CAD build for the part. Positions are in the model's coordinates, mm. A direction names the side the tool comes from. Coordinates: 2 decimals unless noted, no trailing zeros. Order: outer loops, then holes, each group sorted by start corner. A loop starts at its lowest first (then second) coordinate and runs counter-clockwise, first axis right, second up. Notation, with made-up numbers: (23, -35.5) - (58, -35.5) arc R19 cw to (58, -23.5) - close; hole circle Ø8 at (68, -12). An arc over 180 degrees is marked (long way). Write each question's results on one line, items separated by ' | '. Start each with the question number.
Q1. Wall check: probe 1 along X at (y, z) = (-33.5, 0.25); probe 2 along Y at (x, z) = (32, -1); probe 3 along X at (y, z) = (-19.5, -2.5). Give the ranges that are in metal, low to high.
Q2. Which spindle directions (+Z, -Z, +X, -X, +Y, -Y) get a long thin tool onto all of the face, cutting with end or side? Do faces 1 (the cylindrical face through (-18.186, 25.287, 0.296)), 2 (the flat face through (-2, 8, 0)), 3 (the flat face through (10.997, 23, 1)), 4 (the flat face through (-52.003, 23, 1)), 5 (the flat face through (32.247, -7, 1)). Say none if no direction does.
Q3. Band-saw the part on D-D, the plane y = 0. Write the cut outline in (x, z).
Q4. Pull direction X, two halves, no side cores. Call faces 6 (the flat face through (49.497, -13, 0)), 7 (the flat face through (34, -12.503, -2)), 8 (the cylindrical face through (-48.58, 27.496, 0.986)): released by +X, released by -X, zero draft, split by the parting line, or undercut.
Q5. Band-saw the part on B-B, the plane y = -20.5. Write the cut outline in (x, z).
Q6. Band-saw the part on C-C, the plane x = 8.5. Write the cut outline in (y, z), then the cut area to 3 significant figures.
Q7. Band-saw the part on A-A, the plane x = 35. Write the cut outline in (y, z), then the cut area to 3 significant figures.
Q8. Pin check, flat tips, straight feed: P1, Ø1.6, axis at y = 23, z = 1, coming from the -X side; P2, Ø1, axis at x = -6, z = 1.5, coming from the +Y side; P3, Ø1.5, axis at x = -20.5, z = 0.5, coming from the -Y side. Stop position of each tip, or through.
Autodesk Inventor part; units mm, degrees
ref_plane "Work Plane1" through (0, 0, 0) normal (0, 0, 1) x (1, 0, 0)
ref_plane "Work Plane2" through (0, 0, 0) normal (0, 0, 1) x (1, 0, 0)
ref_plane "Work Plane3" through (0, 0, 0) normal (0, 0, 1) x (1, 0, 0)
ref_plane "Work Plane1" through (0, 0, 0) normal (0, 0, 1) x (1, 0, 0)
ref_plane "Work Plane2" through (0, 0, 0) normal (0, 0, 1) x (1, 0, 0)
ref_plane "Work Plane3" through (0, 0, 0) normal (0, 0, 1) x (1, 0, 0)
ref_plane "Work Plane4" through (0, 0, 0) normal (0, 0, 1) x (1, 0, 0)
sketch "Sketch4" plane through (0, 0, 0) normal (0, 0, 1) x (1, 0, 0)
  line L0 (49.4972, -32.0028) -> (22.4972, -32.0028)
  line L1 (22.4972, -32.0028) -> (22.4972, -12.0028)
  line L2 (22.4972, -12.0028) -> (49.4972, -12.0028)
  line L3 (49.4972, -12.0028) -> (49.4972, -1.3028)
  line L4 (49.4972, -1.3028) -> (-34.5028, -1.3028)
  line L5 (-34.5028, -1.3028) -> (-34.5028, 19.2972)
  line L6 (-34.5028, 19.2972) -> (49.4972, 19.2972)
  line L7 (49.4972, 19.2972) -> (49.4972, 23.9972)
  arc A0 (49.4972, 23.9972) -> (42.4972, 23.9972) centre (45.9972, 23.9972) ccw
  line L8 (42.4972, 23.9972) -> (42.4972, 21.9972)
  line L9 (42.4972, 21.9972) -> (17.9972, 21.9972)
  line L10 (17.9972, 21.9972) -> (17.9972, 23.9972)
  arc A1 (17.9972, 23.9972) -> (10.9972, 23.9972) centre (14.4972, 23.9972) ccw
  line L11 (10.9972, 23.9972) -> (10.9972, 21.9972)
  line L12 (10.9972, 21.9972) -> (-13.5028, 21.9972)
  line L13 (-13.5028, 21.9972) -> (-13.5028, 23.9972)
  arc A2 (-13.5028, 23.9972) -> (-20.5028, 23.9972) centre (-17.0028, 23.9972) ccw
  line L14 (-20.5028, 23.9972) -> (-20.5028, 21.9972)
  line L15 (-20.5028, 21.9972) -> (-45.0028, 21.9972)
  line L16 (-45.0028, 21.9972) -> (-45.0028, 23.9972)
  arc A3 (-45.0028, 23.9972) -> (-52.0028, 23.9972) centre (-48.5028, 23.9972) ccw
  line L17 (-52.0028, 23.9972) -> (-52.0028, 21.9972)
  line L18 (-52.0028, 21.9972) -> (-66.5028, 21.9972)
  line L19 (-66.5028, 21.9972) -> (-66.5028, -4.0028)
  line L20 (-66.5028, -4.0028) -> (-20.0885, -4.0028)
  line L21 (-20.0885, -4.0028) -> (-20.0885, -6.0028)
  arc A4 (-20.0885, -6.0028) -> (-13.0885, -6.0028) centre (-16.5885, -6.0028) ccw
  line L22 (-13.0885, -6.0028) -> (-13.0885, -4.0028)
  line L23 (-13.0885, -4.0028) -> (16.4972, -4.0028)
  line L24 (19.4972, -7.0028) -> (19.4972, -36.0028)
  line L25 (22.4972, -39.0028) -> (46.4972, -39.0028)
  line L26 (49.4972, -36.0028) -> (49.4972, -32.0028)
  circle A5 centre (-48.5028, 23.9972) radius 2
  circle A6 centre (-17.0028, 23.9972) radius 2
  circle A7 centre (14.4972, 23.9972) radius 2
  circle A8 centre (45.9972, 23.9972) radius 2
  circle A9 centre (-16.5885, -6.0028) radius 2
  circle A10 centre (45.4972, -8.0028) radius 2
  circle A11 centre (23.4972, -35.0028) radius 2
  circle A12 centre (45.4972, -35.0028) radius 2
  circle A13 centre (23.4972, -8.0028) radius 2
  circle A14 centre (-90.5028, 8.9972) radius 40
  line L27 (49.4972, 19.2972) -> (49.4972, -1.3028)
  line L28 (49.4972, 19.2972) -> (-34.5028, 19.2972)
  line L29 (-34.5028, 19.2972) -> (-34.5028, -1.3028)
  line L30 (49.4972, -1.3028) -> (-34.5028, -1.3028)
  circle A15 centre (-90.5028, 8.9972) radius 40
  line L31 (49.4972, -32.0028) -> (22.4972, -32.0028)
  line L32 (49.4972, -12.0028) -> (49.4972, -32.0028)
  line L33 (22.4972, -12.0028) -> (49.4972, -12.0028)
  line L34 (22.4972, -32.0028) -> (22.4972, -12.0028)
  arc A16 (19.4972, -36.0028) -> (22.4972, -39.0028) centre (22.4972, -36.0028) ccw
  arc A17 (46.4972, -39.0028) -> (49.4972, -36.0028) centre (46.4972, -36.0028) ccw
  arc A18 (19.4972, -7.0028) -> (16.4972, -4.0028) centre (16.4972, -7.0028) ccw
  circle A19 centre (-62.0028, 0.4972) radius 2
  circle A20 centre (-62.0028, 17.4972) radius 2
  circle A21 centre (-56.0028, 8.9972) radius 2
  point P0 (0, 0)
extrude "Extrusion1" add sketch "Sketch4" along normal blind 2 contours L26 A17 L25 A16 L24 A18 L23 L22 A4 L21 L20 A14 L18 L17 A3 L16 L15 L14 A2 L13 L12 L11 A1 L10 L9 L8 A0 L7 L6 L5 L4 L3 L2 L1 L0 | L0 L1 L2 L32 | L4 L5 L6 L27 | L20 L19 L18 A14 | A5 | A6 | A7 | A8 | A9 | A10 | A11 | A12 | A13 | A19 | A20 | A21 picked at (-65.6501, 6.3234)
sketch "Sketch5" plane through (0, 0, 2) normal (0, 0, 1) x (1, 0, 0)
  circle A0 centre (-90.5028, 8.9972) radius 40
  point P0 (0, 0)
extrude "Extrusion2" cut sketch "Sketch5" against normal blind 3
sketch "Sketch6" plane through (0, 0, 0) normal (0, 0, -1) x (-1, 0, 0)
  line L0 (-49.4972, -36.0028) -> (-49.4972, 23.9972)
  line L1 (-19.4972, -7.0028) -> (-19.4972, -36.0028)
  line L2 (13.0885, -4.0028) -> (-16.4972, -4.0028)
  line L3 (-22.4972, -39.0028) -> (-46.4972, -39.0028)
  line L4 (-49.4972, -31.5028) -> (-19.4972, -31.5028)
  line L5 (-19.4972, -31.5028) -> (-19.4972, -12.5028)
  line L6 (-19.4972, -12.5028) -> (-49.4972, -12.5028)
  line L7 (-49.4972, -12.5028) -> (-49.4972, -31.5028)
  line L8 (-49.4972, -31.5028) -> (-19.4972, -12.5028) construction
  line L9 (-19.4972, -31.5028) -> (-49.4972, -12.5028) construction
  line L10 (-19.4972, -7.0028) -> (-19.4972, -36.0028)
  line L11 (-49.4972, -36.0028) -> (-49.4972, 23.9972)
  line L12 (-48.4972, -12.5028) -> (-48.4972, -31.5028)
  point P0 (0, 0)
  point P1 (-19.4972, -21.5028)
  point P2 (-34.4972, -22.0028)
  dimension "d42" = 19
  dimension "d45" = 7.5
  dimension "d47" = 1
extrude "Extrusion3" add sketch "Sketch6" along normal blind 4.1
sketch "Sketch7" plane through (0, 0, 2) normal (0, 0, 1) x (1, 0, 0)
  circle A0 centre (-48.5028, 23.9972) radius 2
  circle A1 centre (-17.0028, 23.9972) radius 2
  circle A2 centre (14.4972, 23.9972) radius 2
  circle A3 centre (45.9972, 23.9972) radius 2
  circle A4 centre (-16.5885, -6.0028) radius 2
  circle A5 centre (23.4972, -35.0028) radius 2
  circle A6 centre (23.4972, -8.0028) radius 2
  circle A7 centre (45.4972, -8.0028) radius 2
  circle A8 centre (45.4972, -35.0028) radius 2
  point P0 (0, 0)
hole "Hole1" at (-16.5885, -6.0028, 2) at (-17.0028, 23.9972, 2) at (-48.5028, 23.9972, 2) at (14.4972, 23.9972, 2) at (45.9972, 23.9972, 2) at (23.4972, -8.0028, 2) at (45.4972, -8.0028, 2) at (45.4972, -35.0028, 2) at (23.4972, -35.0028, 2) direction (0, 0, -1) diameter 3.5 end through all countersink diameter 6.3 countersink angle 90
ref_plane "Work Plane5" through (22.4972, -32.0028, -15) normal (1, 0, 0) x (0, 1, 0)
sketch "Sketch13" plane through (0, 0, 0) normal (0, 0, -1) x (-1, 0, 0)
  line L0 (-42.4972, 21.9972) -> (-17.9972, 21.9972)
  line L1 (-49.4972, -36.0028) -> (-49.4972, 23.9972)
  line L2 (-19.4972, -7.0028) -> (-19.4972, -36.0028)
  point P0 (0, 0)
  point P1 (-34.4972, -6.6528)
  point P2 (-49.4972, -12.0028)
  point P3 (-19.4972, -12.0028)
  dimension "d28" = 28.65
  dimension "d29" = 30
  dimension "d30" = 15
ref_plane "Work Plane6" through (34.4972, -6.6528, 0) normal (1, 0, 0) x (0, 0, -1)
sketch "Sketch14" plane through (34.4972, -6.6528, 0) normal (1, 0, 0) x (0, 0, -1)
  circle A0 centre (1.5, 0) radius 5.5
  line L0 (-2, -29.35) -> (-2, 30.65) construction
  circle A1 centre (1.5, 0) radius 5 construction
  line L1 (-3.5, 0) -> (-3.5, 4.6838) construction
  point P0 (0, 6.6528)
  point P1 (0, 0)
  dimension "d34" = 10
  dimension "d31" = 1.5
  dimension "d32" = 11
extrude "Extrusion7" cut sketch "Sketch14" along normal mid plane 4.5
sketch "Sketch15" plane through (49.4972, -36.0028, 2) normal (1, 0, 0) x (0, 0, -1)
  line L0 (6.1, 4.5) -> (6.1, 23.5)
  line L1 (2, 4.5) -> (6.1, 4.5)
  line L2 (6.1, 23.5) -> (4.1, 23.5)
  line L3 (4.1, 23.5) -> (4.1, 4.5)
  line L4 (4.1, 4.5) -> (6.1, 4.5)
  line L5 (6.1, 4.5) -> (6.1, 23.5)
  point P0 (2, 36.0028)
  point P1 (6.1, 18.5)
  dimension "d48" = 2
extrude "Extrusion8" cut sketch "Sketch15" against normal blind 1
properties part number "support_fourche_partie_capot"
Results below:
1) probe 1: x = 19.5 to 22.6, 24.39 to 44.6, 46.39 to 49.5 | probe 2: y = -31.5 to -12.5 | probe 3: x = 19.5 to 48.5
2) face 1: +Z, -Z | face 2: -Z, +X, -X, +Y | face 3: +Z, -Z, +Y | face 4: +Z, -Z, -X, +Y | face 5: -Z
3) outline: (-51.53, 0) - (49.5, 0) - (49.5, 2) - (-51.53, 2) - close
4) face 6: released by +X | face 7: zero draft | face 8: undercut
5) outline: (19.5, -4.1) - (48.5, -4.1) - (48.5, -2.1) - (49.5, -2.1) - (49.5, 2) - (19.5, 2) - close
6) outline: (-4, 0) - (22, 0) - (22, 2) - (-4, 2) - close | area: 52.0 mm²
7) outline: (-39, 0) - (-31.5, 0) - (-31.5, -4.1) - (-12.5, -4.1) - (-12.5, 0) - (-11.94, 0) arc R5.5 cw to (-10.9, 2) - (-39, 2) - close; (-2.41, 2) arc R5.5 cw to (-1.36, 0) - (22, 0) - (22, 2) - close | area: 180 mm²
8) P1: stops at x = -52 | P2: stops at y = 22 | P3: stops at y = -7.5
